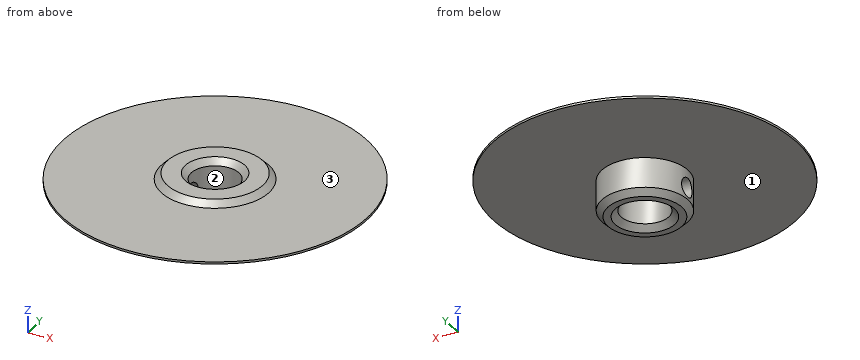
```python
from build123d import *

# Parameters (mm, degrees)
SKETCH_1_R          = 12.7
SKETCH_1_R_2        = 2
EXTRUDE_1_DEPTH     = 0.18
EXTRUDE_START       = 3
SKETCH_2_R          = 3.6
SKETCH_2_R_2        = 2
EXTRUDE_2_DEPTH     = 3
SKETCH_3_R          = 0.8
CUT_EXTRUDE_1_DEPTH = 10
CHAMFER_1_SIZE      = 0.5
SKETCH_4_R          = 4.5
SKETCH_4_R_2        = 2
EXTRUDE_3_DEPTH     = 0.5
CHAMFER_2_SIZE      = 0.5
CHAMFER_3_SIZE      = 0.5


with BuildPart() as part:
    # 草图1 → 凸台-拉伸1 (new body)
    with BuildSketch(Plane.XY):
        with Locations(Location((0, 0, 0), (0, 0, 180))):
            Circle(SKETCH_1_R)
        with Locations(Location((0, 0, 0), (0, 0, 180))):
            Circle(SKETCH_1_R_2, mode=Mode.SUBTRACT)
    extrude(amount=EXTRUDE_1_DEPTH)

    # 草图2 → 凸台-拉伸2 (add)
    with BuildSketch(Plane(origin=(0, 0, 0), x_dir=(-1, 0, 0), z_dir=(0, 0, -1)).offset(EXTRUDE_START)):
        with Locations(Location((0, 0, 0), (0, 0, 180))):
            Circle(SKETCH_2_R)
        Circle(SKETCH_2_R_2, mode=Mode.SUBTRACT)
    extrude(amount=-EXTRUDE_2_DEPTH)

    # 草图3 → 切除-拉伸1 (cut)
    with BuildSketch(Plane(origin=(0, 0, 0), x_dir=(0, 0, -1), z_dir=(1, 0, 0))):
        with Locations((1.5, 0)):
            Circle(SKETCH_3_R)
    extrude(amount=-CUT_EXTRUDE_1_DEPTH, mode=Mode.SUBTRACT)

    # 倒角1
    chamfer_1_edges = [part.edges().sort_by_distance(p)[0] for p in [
        (-3.6, 0, -3),
        (2, 0, -3),
    ]]
    chamfer(chamfer_1_edges, length=CHAMFER_1_SIZE)

    # 草图4 → 凸台-拉伸3 (add)
    with BuildSketch(Plane.XY.offset(0.18)):
        Circle(SKETCH_4_R)
        with Locations(Location((0, 0, 0), (0, 0, 180))):
            Circle(SKETCH_4_R_2, mode=Mode.SUBTRACT)
    extrude(amount=EXTRUDE_3_DEPTH)

    # 倒角2
    chamfer_2_edges = [part.edges().sort_by_distance(p)[0] for p in [
        (-4.5, 0, 0.68),
    ]]
    chamfer(chamfer_2_edges, length=CHAMFER_2_SIZE - 0.0001)  # a hair under: the kernel refuses the full size

    # 倒角3
    chamfer_3_edges = [part.edges().sort_by_distance(p)[0] for p in [
        (2, 0, 0.68),
    ]]
    chamfer(chamfer_3_edges, length=CHAMFER_3_SIZE)


solid = part.part
```
Model file for the job. Use its own axes, mm. Face numbers are marked on the shaded views. A direction names the side the tool comes from. Round coordinates to 2 decimals unless told otherwise and drop trailing zeros. Write each loop counter-clockwise with the first axis right and the second up, starting at its lowest first coordinate (ties: lowest second). Pieces come first, ordered by that corner, then holes. Notation, with made-up numbers: (56, 44.5) - (114, 44.5) arc R28 ccw to (114, 71.5) - close; hole circle Ø2 at (81, 56.5). An arc over 180 degrees is marked (long way). Use CSV: the item, a comma, the result in double quotes. Start each with the question number.
Item 1: Tool access for the marked faces 1, 2 and 3: list every direction of +Z, -Z, +X, -X, +Y, -Y with a clear straight run to the whole face (end or side of a thin tool).
Item 2: Pin check, flat tips, straight feed: P1, Ø4, axis at x = 9, y = -8.5, coming from the -Z side; P2, Ø1.5, axis at y = -9.5, z = -2.5, coming from the +X side; P3, Ø1.8, axis at y = 0, z = -1.5, coming from the +X side. Stop position of each tip, or through.
Item 3: Band-saw the part on A-A (y = 0). State how many separate pieces and enclosed holes the cut face has, and give its area (3 significant figures).
Item 4: Drill centre lines: L1, parallel to Y at x = 0, z = -0.65; L2, parallel to Z at x = -11.25, y = -5.5; L3, parallel to Y at x = -2.2, z = -1.5. Where is each one in solid material? Low to high. Write a range as [from, to].
Item 5: Band-saw the part on C-C (z = -1.5). Write the cut outline in (x, y), and give its area (3 significant figures).
Item 6: Band-saw the part on D-D (x = -9). Write the cut outline in (y, z), and give its area (3 significant figures).
Checked values:
1,face 1,"-Z"
1,face 2,"+Z, -Z"
1,face 3,"+Z"
2,P1,"stops at z = 0"
2,P2,"passes through"
2,P3,"stops at x = 3.6"
3,separate pieces,"3"
3,enclosed holes,"0"
3,area,"12.4 mm²"
4,L1,"y = [-3.6, -2], [2, 3.6]"
4,L2,"z = [0, 0.18]"
4,L3,"y = [-2.85, -0.8], [0.8, 2.85]"
5,outline,"(-3.51, -0.8) arc R3.6 ccw (long way) to (-3.51, 0.8) - (-1.83, 0.8) arc R2 cw (long way) to (-1.83, -0.8) - close"
5,area,"25.5 mm²"
6,outline,"(-8.96, 0) - (8.96, 0) - (8.96, 0.18) - (-8.96, 0.18) - close"
6,area,"3.23 mm²"
